The model under review builds one solid part; all positions refer to its coordinate system, in mm. Give positions to 0.01 mm unless a question says otherwise; leave off trailing zeros. Loops run counter-clockwise (first coordinate to the right, second up) from the corner with the lowest first, then second, coordinate; pieces in that order, holes last. Notation, with made-up numbers: (24.5, 85) - (59.5, 85) arc R18 ccw to (59.5, 94) - close; hole circle Ø8 at (-6, 79.25). An arc over 180 degrees is marked (long way). Return JSON: item names as keys, results as strings. Group by question number.
Autodesk Fusion 360 part; units mm, degrees
sketch "スケッチ1" plane through (0, 0, 0) normal (0, 0, 1) x (1, 0, 0)
  line L0 (2.5, 186) -> (-92.5, 186)
  line L1 (-92.5, 186) -> (-92.5, -186)
  line L2 (-92.5, -186) -> (2.5, -186)
  line L3 (92.5, 0) -> (92.5, 180)
  line L4 (89.5161, 180) -> (-92.5, -186) construction
  line L5 (-92.5, 186) -> (46.8836, -94.274) construction
  line L6 (2.5, 186) -> (2.5, 180)
  line L7 (2.5, 180) -> (92.5, 180)
  line L8 (-92.5, -186) -> (2.5, -186) construction
  line L9 (92.5, 0) -> (2.5, -186)
  dimension "d2" = 372
  dimension "d5" = 95
extrude "押し出し1" add sketch "スケッチ1" along normal blind 6
sketch "スケッチ2" plane through (0, 0, 6) normal (0, 0, 1) x (-1, 0, 0)
  line L0 (-2.5, -186) -> (92.5, -186)
  line L1 (92.5, -186) -> (92.5, 186)
  line L2 (92.5, 186) -> (-2.5, 186)
  line L3 (-2.5, 186) -> (-92.5, 0)
  line L4 (-92.5, 0) -> (-92.5, -180)
  line L5 (-92.5, -180) -> (-2.5, -180)
  line L6 (-2.5, -180) -> (-2.5, -186)
  line L7 (-92.5, -180) -> (-52.5, -180) construction
  line L8 (-52.5, -180) -> (-52.5, -130) construction
  line L9 (-52.5, -130) -> (-92.5, -130) construction
  line L10 (-92.5, -130) -> (-92.5, -180) construction
  line L11 (-52.5, -130) -> (-52.5, -70) construction
  point P0 (-52.5, -130)
  point P1 (-52.5, -70)
  dimension "d9" = 40
  dimension "d10" = 50
  dimension "d11" = 60
hole "穴1" at (52.5, 130, 6) at (52.5, 70, 6) direction (0, 0, -1) diameter 18 end through all
chamfer "面取り1" distance 30 angle 45 2 edges at (-92.5, -186, 3) (-92.5, 186, 3)
equation "d5 = 30 mm + 65 mm"
Item 1: Take a section at D-D (x = 22). State the section outline as (y, z) points, then the cut area to 3 significant figures.
Item 2: Mouldability with a two-part tool opening along X and no side actions: class faces 1 (the face through (-1, 3, 0)), 2 (the face through (48.13, -91.7, 2.96)), 3 (the face through (49.797, 121.416, 2.958)), 4 (the face through (49.797, 61.416, 2.958)) as +X half, -X half, draft (parallel to the pull), parting line (faces both ways), or undercut.
Item 3: Take a section at A-A (z = 1.6). State the section outline as (x, y) points, then the cut area to 3 significant figures.
Item 4: Take a section at B-B (y = 130). State the section outline as (x, z) points, then the cut area to 3 significant figures.
Item 5: For P1, Ø3, axis at x = 63.5, z = 3.5, coming from the +Y side, flat-tipped, find the tip position at first contact; note if it passes through.
Item 6: For L1, parallel to X at y = 70, z = 2.2; L2, parallel to Y at x = 52.5, z = 3.6; L3, parallel to X at y = -28, z = 3.45, list the stretches that pass through material, from the lowest coordinate up. Write a range as from..to.
Item 7: Take a section at C-C (x = 52.5). State the section outline as (y, z) points.
Check sheet entries:
{
 "1": {"outline": "(-145.7, 0) - (180, 0) - (180, 6) - (-145.7, 6) - close", "area": "1,950 mm^2"},
 "2": {"face 1": "draft", "face 2": "+X half", "face 3": "undercut", "face 4": "undercut"},
 "3": {"outline": "(-92.5, -156) - (-62.5, -186) - (2.5, -186) - (92.5, 0) - (92.5, 180) - (2.5, 180) - (2.5, 186) - (-62.5, 186) - (-92.5, 156) - close; hole circle Ø18 at (52.5, 70); hole circle Ø18 at (52.5, 130)", "area": "58,500 mm^2"},
 "4": {"outline": "(-92.5, 0) - (43.5, 0) - (43.5, 6) - (-92.5, 6) - close; (61.5, 0) - (92.5, 0) - (92.5, 6) - (61.5, 6) - close", "area": "1,000 mm^2"},
 "5": {"P1": "stops at y = 180"},
 "6": {"L1": "x = -92.5..43.5, 61.5..92.5", "L2": "y = -82.67..61, 79..121, 139..180", "L3": "x = -92.5..78.95"},
 "7": {"outline": "(-82.67, 0) - (61, 0) - (61, 6) - (-82.67, 6) - close; (79, 0) - (121, 0) - (121, 6) - (79, 6) - close; (139, 0) - (180, 0) - (180, 6) - (139, 6) - close"}
}
